Part model, mm, in its own coordinate system. Face numbers are marked on the shaded views. A direction names the side the tool comes from. Round coordinates to 2 decimals unless told otherwise and drop trailing zeros. Write each loop counter-clockwise with the first axis right and the second up, starting at its lowest first coordinate (ties: lowest second). Pieces come first, ordered by that corner, then holes.
1) Flat gauge pins, fed straight in: pin 1 (25 mm diameter, centred on x = 48.5, y = 69.5, fed in from -Z); pin 2 (17 mm diameter, centred on x = -48.5, y = 25.5, fed in from -Z). Where does each tip first touch, or does it go through?
2) Drill centre lines: L1, parallel to X at y = 4, z = 1.3; L2, parallel to X at y = 82, z = 1; L3, parallel to Y at x = -15.5, z = 0.8. Where is each one in solid material? Low to high.
3) Saw through at C-C on x = 3.5. Write the cut outline in (y, z).
4) Saw through at D-D on y = 56.5. Write the cut outline in (x, z), and give its area (3 significant figures).
5) Saw through at A-A on y = 4. Write the cut outline in (x, z).
6) Pull direction X, two halves, no side cores. Call the marked faces 3, 4 and 5: +X half, -X half, draft (parallel to the pull), parting line (faces both ways), or undercut.
7) Which spindle directions (+Z, -Z, +X, -X, +Y, -Y) get a long thin tool onto all of the face, cutting with end or side? Do the marked faces 1 and 2. Say none if no direction does.
8) Saw through at B-B on y = -16. Write the cut outline in (x, z), and give its area (3 significant figures).
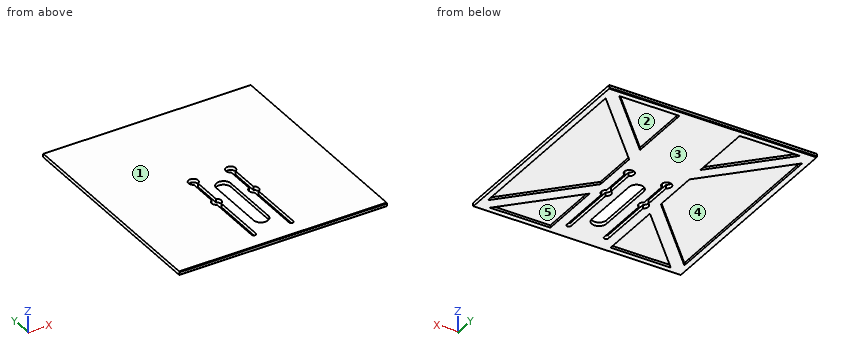
Autodesk Fusion 360 part; units mm, degrees
sketch "Sketch1" plane through (0, 0, 0) normal (0, 0, 1) x (1, 0, 0)
  line L0 (86.5, 91.5) -> (-86.5, 91.5)
  line L1 (-86.5, 91.5) -> (-86.5, -91.5)
  line L2 (-86.5, -91.5) -> (86.5, -91.5)
  line L3 (86.5, -91.5) -> (86.5, 91.5)
  line L4 (86.5, 91.5) -> (-86.5, -91.5) construction
  line L5 (-86.5, 91.5) -> (86.5, -91.5) construction
  line L6 (0, -91.5) -> (0, -61.5)
  line L7 (15.5, -77) -> (-15.5, -77)
  line L8 (-15.5, -77) -> (-15.5, -46)
  line L9 (-15.5, -46) -> (15.5, -46)
  line L10 (15.5, -46) -> (15.5, -77)
  line L11 (15.5, -77) -> (-15.5, -46) construction
  line L12 (-15.5, -77) -> (15.5, -46) construction
  circle A0 centre (-15.5, -77) radius 1.75
  circle A1 centre (-15.5, -46) radius 1.75
  circle A2 centre (15.5, -46) radius 1.75
  circle A3 centre (15.5, -77) radius 1.75
  line L13 (0, -61.5) -> (0, -11.5)
  line L14 (15.5, -27) -> (-15.5, -27)
  line L15 (-15.5, -27) -> (-15.5, 4)
  line L16 (-15.5, 4) -> (15.5, 4)
  line L17 (15.5, 4) -> (15.5, -27)
  line L18 (15.5, -27) -> (-15.5, 4) construction
  line L19 (-15.5, -27) -> (15.5, 4) construction
  circle A4 centre (-15.5, 4) radius 1.75
  circle A5 centre (15.5, 4) radius 1.75
  circle A6 centre (15.5, -27) radius 1.75
  circle A7 centre (-15.5, -27) radius 1.75
  circle A8 centre (-15.5, 4) radius 4
  circle A9 centre (15.5, 4) radius 4
  circle A10 centre (0, -61.5) radius 6
  circle A11 centre (0, -11.5) radius 6
  line L20 (13.75, 4) -> (17.25, 4)
  line L21 (17.25, 4) -> (17.25, -77)
  line L22 (17.25, -77) -> (13.75, -77)
  line L23 (13.75, -77) -> (13.75, 4)
  line L24 (-13.75, 4) -> (-17.25, 4)
  line L25 (-17.25, 4) -> (-17.25, -77)
  line L26 (-17.25, -77) -> (-13.75, -77)
  line L27 (-13.75, -77) -> (-13.75, 4)
  line L28 (-6, -11.5) -> (6, -11.5)
  line L29 (6, -11.5) -> (6, -61.5)
  line L30 (6, -61.5) -> (-6, -61.5)
  line L31 (-6, -61.5) -> (-6, -11.5)
  line L32 (25, -91.5) -> (-25, -91.5)
  line L33 (-25, -91.5) -> (-25, 91.5)
  line L34 (-25, 91.5) -> (25, 91.5)
  line L35 (25, 91.5) -> (25, -91.5)
  line L36 (25, -91.5) -> (-25, 91.5) construction
  line L37 (-25, -91.5) -> (25, 91.5) construction
  line L38 (-86.5, -91.5) -> (86.5, 91.5)
  line L39 (86.5, 91.5) -> (82.8666, 94.9349)
  line L40 (82.8666, 94.9349) -> (-90.1334, -88.0651)
  line L41 (-90.1334, -88.0651) -> (-86.5, -91.5)
  line L42 (-86.5, -91.5) -> (86.5, 91.5)
  line L43 (86.5, 91.5) -> (90.1334, 88.0651)
  line L44 (90.1334, 88.0651) -> (-82.8666, -94.9349)
  line L45 (-82.8666, -94.9349) -> (-86.5, -91.5)
  line L46 (86.5, -91.5) -> (-86.5, 91.5)
  line L47 (-86.5, 91.5) -> (-82.8666, 94.9349)
  line L48 (-82.8666, 94.9349) -> (90.1334, -88.0651)
  line L49 (90.1334, -88.0651) -> (86.5, -91.5)
  line L50 (86.5, -91.5) -> (-86.5, 91.5)
  line L51 (-86.5, 91.5) -> (-90.1334, 88.0651)
  line L52 (-90.1334, 88.0651) -> (82.8666, -94.9349)
  line L53 (82.8666, -94.9349) -> (86.5, -91.5)
  line L54 (81.5, -86.5) -> (-81.5, -86.5)
  line L55 (-81.5, -86.5) -> (-81.5, 86.5)
  line L56 (-81.5, 86.5) -> (81.5, 86.5)
  line L57 (81.5, 86.5) -> (81.5, -86.5)
  line L58 (81.5, -86.5) -> (-81.5, 86.5) construction
  line L59 (-81.5, -86.5) -> (81.5, 86.5) construction
  circle A12 centre (-15.5, -27) radius 4
  circle A13 centre (15.5, -27) radius 4
  point P0 (0, -91.5)
  point P1 (0, -61.5)
  point P2 (0, -11.5)
  dimension "d1" = 173
  dimension "d2" = 183
  dimension "d3" = 30
  dimension "d4" = 31
  dimension "d5" = 31
  dimension "d6" = 3.5
  dimension "d7" = 3.5
  dimension "d8" = 3.5
  dimension "d9" = 3.5
  dimension "d10" = 50
  dimension "d11" = 31
  dimension "d12" = 31
  dimension "d13" = 3.5
  dimension "d14" = 3.5
  dimension "d15" = 3.5
  dimension "d16" = 3.5
  dimension "d17" = 8
  dimension "d18" = 8
  dimension "d19" = 12
  dimension "d20" = 12
  dimension "d21" = 3.5
  dimension "d22" = 3.5
  dimension "d31" = 50
  dimension "d32" = 5
  dimension "d33" = 5
  dimension "d34" = 5
  dimension "d35" = 5
  dimension "d36" = 163
  dimension "d37" = 173
  dimension "d42" = 8
  dimension "d43" = 8
extrude "Extrude1" add sketch "Sketch1" along normal blind 3 contours L0 L33 L34 L35 L56 | L0 L35 L40 L56 | L0 L33 L48 L56 | L0 L38 L40 L42 L56 L57 | L35 L40 L56 | L33 L35 L40 L48 L56 | L0 L46 L48 L50 L55 L56 | L33 L48 L56 | L3 L38 L42 L44 L57 | L35 L38 L40 L42 L56 L57 | L16 L35 L38 L40 L42 L48 | L1 L46 L50 L52 L55 | L33 L46 L48 L50 L55 L56 | L16 L33 L40 L46 L48 L50 | L3 L44 L48 L57 | L35 L38 L42 L44 L57 | L16 A9 L35 L38 L42 L44 | L16 L40 L48 | L1 L40 L52 L55 | L33 L46 L50 L52 L55 | L16 A8 L33 L46 L50 L52 | L3 L46 L48 L50 L57 | L35 L44 L48 L57 | A9 L21 L35 L44 L48 | L16 L38 L42 L48 | L16 L38 L42 L44 L48 | L16 L40 L46 L50 | L16 L38 L40 L42 L46 L48 L50 | L1 L38 L40 L42 L55 | L33 L40 L52 L55 | A8 L25 L33 L40 L52 | L16 L40 L46 L50 L52 | L2 L46 L50 L52 L54 L57 | L35 L46 L48 L50 L57 | L21 L35 L46 L48 L50 | L16 A9 L44 | L16 A9 L23 L44 L48 | L38 L42 L44 L46 L48 L50 | L38 L40 L42 L46 L50 L52 | L2 L38 L42 L44 L54 L55 | L33 L38 L40 L42 L55 | L25 L33 L38 L40 L42 | L16 A8 L27 L40 L52 | L16 A8 L52 | L2 L35 L52 L54 | L35 L46 L50 L52 L54 L57 | L21 L35 L46 L50 L52 A13 | L23 L44 L46 L48 L50 | A11 L38 L42 L44 L46 L50 L52 | L27 L38 L40 L42 L52 | L2 L33 L44 L54 | L33 L38 L42 L44 L54 L55 | L25 L33 L38 L42 L44 A12 | L2 L6 L32 L35 L54 | L35 L52 L54 | L6 L7 A3 L21 L35 L52 L54 A13 | A11 L23 L29 L44 L46 L50 L52 | A11 L27 L31 L38 L42 L44 L52 | L2 L6 L32 L33 L54 | L33 L44 L54 | L6 L7 A0 L25 L33 L44 L54 A12 | L21 L52 A13 | L21 L52 A13 | L25 L44 A12 | L25 L44 A12 | L14 L23 L29 L52 A13 | L14 L27 L31 L44 A12 | L6 L7 L9 A10 L27 L31 | L6 L7 L9 A10 L23 L29 | L14 L23 A13 | L9 L14 L23 L29 A13 | L14 L23 A13 | L14 L27 A12 | L9 L14 L27 L31 A12 | L14 L27 A12
chamfer "Chamfer1" distance 0.5 angle 45 2 edges at (0, -91.5, 3) (0, -91.5, 0)
chamfer "Chamfer2" distance 0.5 angle 45 2 edges at (0, 91.5, 3) (0, 91.5, 0)
extrude "Extrude2" cut 1 faces at (86.5, 30.3333, 2) along direction (-1, 0, 0) blind 0.5
extrude "Extrude3" cut 1 faces at (-86.5, -30.3333, 2) along direction (1, 0, 0) blind 0.5
extrude "Extrude5" cut sketch "Sketch1" along normal blind 2 contours L35 L40 L56 | L33 L48 L56 | L35 L44 L48 L57 | L33 L40 L52 L55 | L35 L52 L54 | L33 L44 L54
extrude "Extrude6" cut sketch "Sketch1" along normal blind 3 contours L21 L52 A13 | L21 L52 A13 | L17 L21 L52 A13 | L25 L44 A12 | L25 L44 A12 | L15 L25 L44 A12 | L17 A6 L21 L52 | A6 L21 L23 A13 | L17 L52 A13 | L15 A7 L25 L44 | A7 L25 L27 A12 | L15 L44 A12 | L14 L17 A6 | L17 A6 L23 L52 A13 | L14 L23 A13 | L14 L23 A13 | L14 L27 A12 | L15 A7 L27 L44 A12 | L14 L15 A7 | L14 L27 A12 | L14 L17 A6 | L14 L15 A7
equation "d36 = 173.000 mm - 10 mm"
equation "d37 = 183.000 mm - 10 mm"
Completed:
1. pin 1: stops at z = 0
1. pin 2: stops at z = 2
2. L1: x = -86 to -81.5, -25 to -19.5, -11.5 to 11.5, 19.5 to 25, 81.5 to 86
2. L2: x = -86 to -70.64, -25 to 25, 70.64 to 86
2. L3: y = -91.5 to -78.75, 8 to 91.5
3. outline: (-91.5, 0.5) - (-91, 0) - (-66.37, 0) - (-66.37, 3) - (-91, 3) - (-91.5, 2.5) - close; (-6.63, 0) - (91, 0) - (91.5, 0.5) - (91.5, 2.5) - (91, 3) - (-6.63, 3) - close
4. outline: (-86, 0) - (-81.5, 0) - (-81.5, 2) - (-60.29, 2) - (-60.29, 0) - (-46.53, 0) - (-46.53, 2) - (-25, 2) - (-25, 0) - (25, 0) - (25, 2) - (46.53, 2) - (46.53, 0) - (60.29, 0) - (60.29, 2) - (81.5, 2) - (81.5, 0) - (86, 0) - (86, 3) - (-86, 3) - close
4. area: 345 mm2
5. outline: (-86, 0) - (-81.5, 0) - (-81.5, 2) - (-25, 2) - (-25, 0) - (-19.5, 0) - (-19.5, 3) - (-86, 3) - close; (-11.5, 0) - (11.5, 0) - (11.5, 3) - (-11.5, 3) - close; (19.5, 0) - (25, 0) - (25, 2) - (81.5, 2) - (81.5, 0) - (86, 0) - (86, 3) - (19.5, 3) - close
6. face 3: draft
6. face 4: undercut
6. face 5: undercut
7. face 1: +Z, +X, -X, +Y, -Y
7. face 2: -Z
8. outline: (-86, 0) - (-81.5, 0) - (-81.5, 2) - (-25, 2) - (-25, 0) - (-17.25, 0) - (-17.25, 3) - (-86, 3) - close; (-13.75, 0) - (-6, 0) - (-6, 3) - (-13.75, 3) - close; (6, 0) - (13.75, 0) - (13.75, 3) - (6, 3) - close; (17.25, 0) - (25, 0) - (25, 2) - (81.5, 2) - (81.5, 0) - (86, 0) - (86, 3) - (17.25, 3) - close
8. area: 233 mm2
